For this review, use the dimensioned drawing (mm, ordinates from the lowest corner) and the shaded views. A direction names the side the tool comes from. Coordinates: 2 decimals unless noted, no trailing zeros. Loops run counter-clockwise (first coordinate to the right, second up) from the corner with the lowest first, then second, coordinate; pieces in that order, holes last.
1. To check wall thickness, follow probe 1 along Z at (x, y) = (17.5, 3); probe 2 along Y at (x, z) = (19, 3); probe 3 along X at (y, z) = (11, 7.75) (1 decimal). State the ranges of each line that lie inside material, in increasing order.
2. Machinability: for the marked faces 1, 2, 3 and 4, which of the approach directions +Z, -Z, +X, -X, +Y, -Y give a long, thin tool a straight path to every point of the face, cutting with its end or side? Answer none if there is none.
3. Take a section at B-B, the plane x = 4.5. State the section outline as (y, z) points.
4. Take a section at C-C, the plane z = 1.25. State the section outline as (x, y) points (1 decimal).
5. Clearance check with flat-ended pins moving along their axes: P1, Ø1.5, axis at y = 3, z = 9, coming from the +X side; P2, Ø7, axis at x = 3.5, z = 6.5, coming from the +Y side; P3, Ø1.8, axis at x = 9, y = 7.5, coming from the +Z side. State where each tip first meets the part, or that it passes through.
6. Take a section at D-D, the plane y = 11. State the section outline as (x, z) points.
7. Take a section at A-A, the plane y = 5.75. State the section outline as (x, z) points (1 decimal), then the cut area to 3 significant figures.
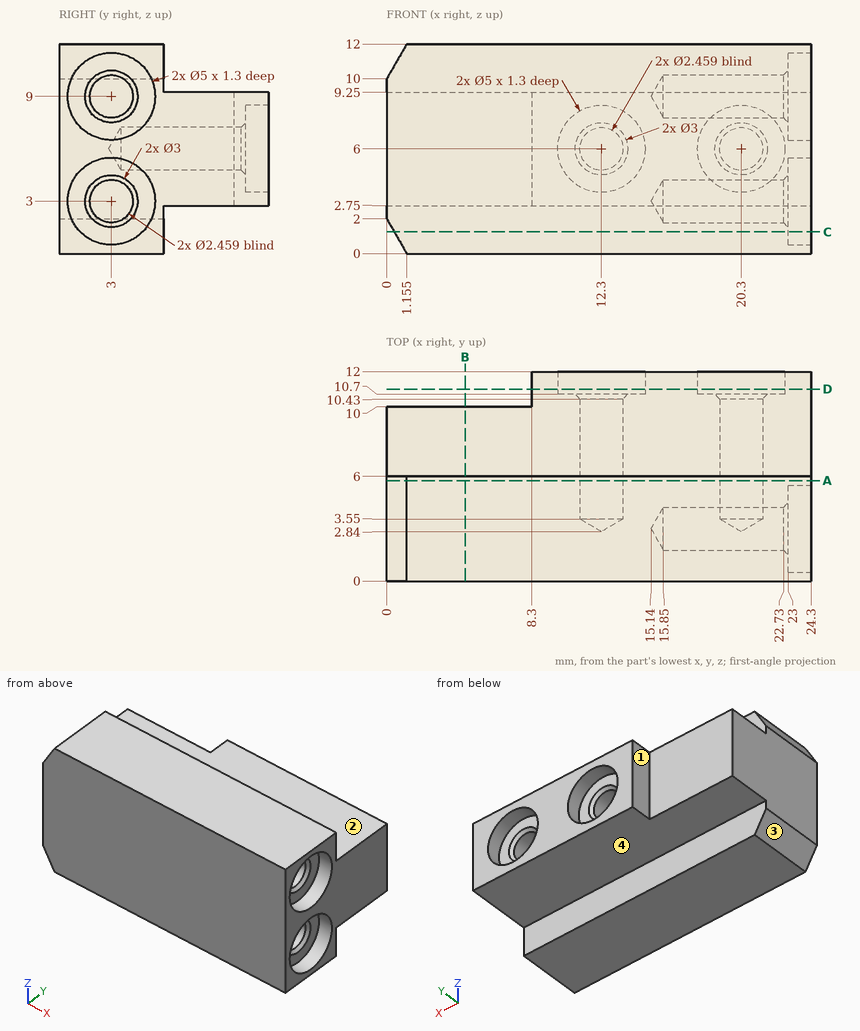
Results list:
1. probe 1: z = 0 to 1.77, 4.23 to 7.77, 10.23 to 12
1. probe 2: y = 0 to 1.77, 4.23 to 12
1. probe 3: x = 8.3 to 10.5, 14.1 to 18.5, 22.1 to 24.3
2. face 1: +Z, -Z, -X, +Y
2. face 2: +Z, +X, -X, +Y
2. face 3: -Z, -X, +Y, -Y
2. face 4: -Z, +X, -X, +Y
3. outline: (0, 0) - (6, 0) - (6, 2.75) - (10, 2.75) - (10, 9.25) - (6, 9.25) - (6, 12) - (0, 12) - close
4. outline: (0.4, 0) - (24.3, 0) - (24.3, 1.2) - (23, 1.2) - (23, 4.8) - (24.3, 4.8) - (24.3, 6) - (0.4, 6) - close
5. P1: stops at x = 15.57
5. P2: stops at y = 10
5. P3: stops at z = 9.25
6. outline: (8.3, 2.75) - (24.3, 2.75) - (24.3, 9.25) - (8.3, 9.25) - close; hole circle Ø5 at (12.3, 6); hole circle Ø5 at (20.3, 6)
7. outline: (0, 2) - (1.2, 0) - (24.3, 0) - (24.3, 12) - (1.2, 12) - (0, 10) - close; hole circle Ø2.5 at (12.3, 6); hole circle Ø2.5 at (20.3, 6)
7. area: 280 mm2
